Source: CAD feature listing. Evaluate the final solid. Frame: model axes, mm. A direction names the side the tool comes from. Round coordinates to 2 decimals unless told otherwise and drop trailing zeros. Order: outer loops, then holes, each group sorted by start corner. A loop starts at its lowest first (then second) coordinate and runs counter-clockwise, first axis right, second up. Notation, with made-up numbers: M 68.25,5.25 L 104.25,5.25 A29 ccw 104.25,31.25 Z; hole C 51.25,32.5 d3. An arc over 180 degrees is marked long. Use one line per item in the form item = value. Start each with the question number.
Q1. Material intervals for probe 1 along Z at (x, y) = (25, 55); probe 2 along X at (y, z) = (99.5, 2.45); probe 3 along Y at (x, z) = (29, 5), sorted ascending.
Q2. Section C-C (z = 4.25). Return the cut outline in (x, y), plus the area to 3 significant figures.
Q3. Contact query for flat-ended pins moving along their axis: pin 1 (1.5 mm diameter, centred on y = 271, z = 2, fed in from -X); pin 2 (0.9 mm diameter, centred on x = 1.5, z = 1.5, fed in from +Y); pin 3 (3.5 mm diameter, centred on x = 1, z = 1.5, fed in from -Y); pin 4 (1 mm diameter, centred on y = 130.5, z = 4.5, fed in from -X). Output: stop coordinate, or through.
Q4. Section B-B (x = 37.5). Return the cut outline in (y, z).
Q5. Section D-D (y = 68). Return the cut outline in (x, z).
Q6. Section A-A (y = 275). Return the cut outline in (x, z).
Q7. Reachability of faces 1 (the cylindrical face through (8.555, 9.021, 1.521)), 2 (the cylindrical face through (44.985, 29.34, 4.479)) from +Z, -Z, +X, -X, +Y, -Y: full face, straight path, thin tool, end or side. Return the list, or none.
from build123d import *

# Parameters (mm, degrees)
ESQUISSE1_W             = 60
ESQUISSE1_H             = 380
BOSS_EXTRU_1_DEPTH      = 3
CONG_1_R                = 30
ESQUISSE2_W             = 3
ESQUISSE2_H             = 25
ENL_V_MAT_EXTRU_1_DEPTH = 3
ESQUISSE3_R             = 15
BOSS_EXTRU_2_DEPTH      = 3
ESQUISSE4_W             = 3
ESQUISSE4_H             = 25
ENL_V_MAT_EXTRU_2_DEPTH = 3


with BuildPart() as part:
    # Esquisse1 → Boss.-Extru.1 (new body)
    with BuildSketch(Plane.XY):
        with Locations((30, 190)):
            Rectangle(ESQUISSE1_W, ESQUISSE1_H)
    extrude(amount=BOSS_EXTRU_1_DEPTH)

    # Congé1
    cong_1_edges = [part.edges().sort_by_distance(p)[0] for p in [
        (0, 0, 1.5),
        (60, 0, 1.5),
    ]]
    fillet(cong_1_edges, radius=CONG_1_R - 0.0001)  # a hair under: the kernel refuses the full size

    # Esquisse2 → Enlèv. mat.-Extru.1 (cut)
    with BuildSketch(Plane.XY.offset(3)):
        with Locations((1.5, 367.5)):
            Rectangle(ESQUISSE2_W, ESQUISSE2_H)
        with Locations((1.5, 317.5)):
            Rectangle(ESQUISSE2_W, ESQUISSE2_H)
        with Locations((1.5, 267.5)):
            Rectangle(ESQUISSE2_W, ESQUISSE2_H)
    extrude(amount=-ENL_V_MAT_EXTRU_1_DEPTH, mode=Mode.SUBTRACT)

    # Esquisse3 → Boss.-Extru.2 (add)
    with BuildSketch(Plane.XY.offset(3)):
        with Locations(Location((30, 30, 0), (0, 0, 180))):
            Circle(ESQUISSE3_R)
    extrude(amount=BOSS_EXTRU_2_DEPTH)

    # Esquisse4 → Enlèv. mat.-Extru.2 (cut)
    with BuildSketch(Plane.XY.offset(3)):
        with Locations((1.5, 42.5)):
            Rectangle(ESQUISSE4_W, ESQUISSE4_H)
        with Locations((1.5, 92.5)):
            Rectangle(ESQUISSE4_W, ESQUISSE4_H)
    extrude(amount=-ENL_V_MAT_EXTRU_2_DEPTH, mode=Mode.SUBTRACT)


solid = part.part
Results list:
q1.probe_1 = 0 to 3
q1.probe_2 = 3 to 60
q1.probe_3 = 15.03 to 44.97
q2.outline = C 30,30 d30
q2.area = 707 mm2
q3.pin_1 = 3
q3.pin_2 = 355
q3.pin_3 = 17.45
q3.pin_4 = through
q4.outline = M 0.95,0 L 380,0 L 380,3 L 42.99,3 L 42.99,6 L 17.01,6 L 17.01,3 L 0.95,3 Z
q5.outline = M 0,0 L 60,0 L 60,3 L 0,3 Z
q6.outline = M 3,0 L 60,0 L 60,3 L 3,3 Z
q7.face_1 = +Z, -Z, -X, -Y
q7.face_2 = +Z
